For this review, use the dimensioned drawing (mm, ordinates from the lowest corner) and the shaded views. Coordinates: 2 decimals unless noted, no trailing zeros. Order: outer loops, then holes, each group sorted by start corner. A loop starts at its lowest first (then second) coordinate and runs counter-clockwise, first axis right, second up. Notation, with made-up numbers: M 63,20 L 101,20 A19 ccw 101,54 Z; hole C -26,42 d11. An arc over 180 degrees is marked long. Use one line per item in the form item = value. Start each with the question number.
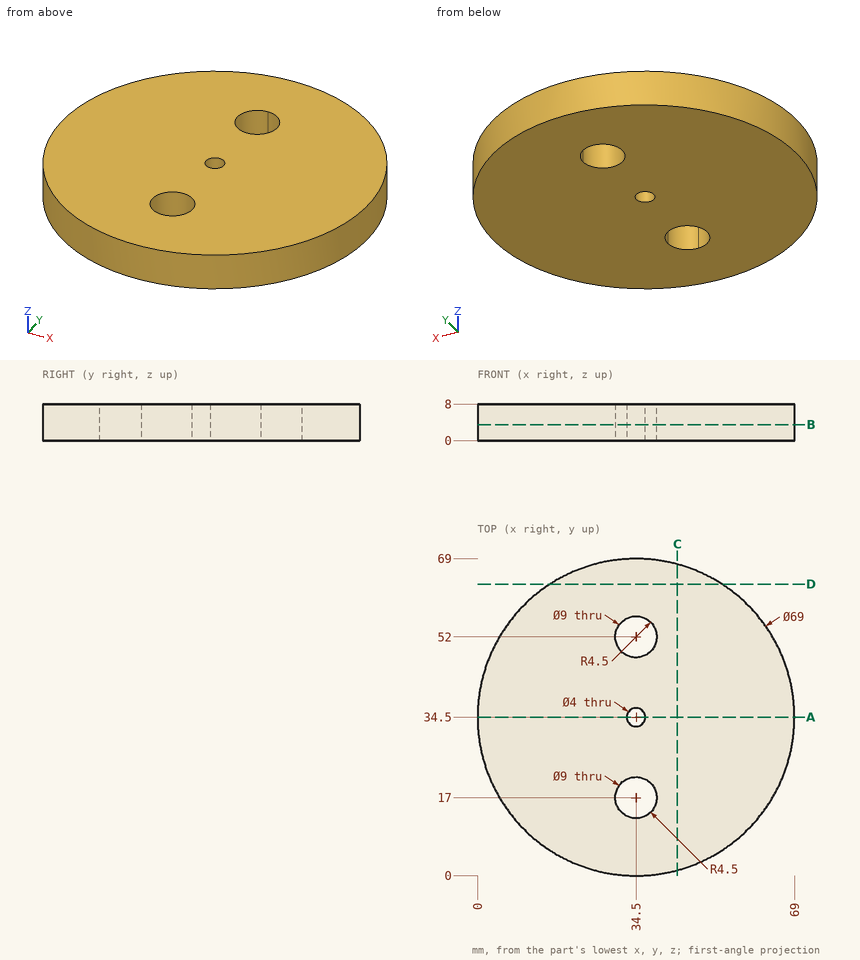
1. Consider section A-A, the plane y = 34.5. Write out the cut boundary in (x, z), plus the area to 3 significant figures.
2. To check wall thickness, follow line 1 (Y direction, x = 34.5, z = 3.75); line 2 (Y direction, x = 37.5, z = 5.5); line 3 (X direction, y = 17, z = 2.75). State the ranges of each line that lie inside material, in increasing order.
3. Consider section C-C, the plane x = 43.5. Write out the cut boundary in (y, z), plus the area to 3 significant figures.
4. Consider section D-D, the plane y = 63.5. Write out the cut boundary in (x, z).
5. Consider section B-B, the plane z = 3.5. Write out the cut boundary in (x, y).
6. For pin 1 Ø3 at (x, z) = (50, 1.5) entering from +Y; pin 2 Ø2 at (x, z) = (51, 1) entering from +Y; pin 3 Ø3 at (x, y) = (34.5, 34.5) entering from +Z; pin 4 Ø4 at (y, z) = (60.5, 4.5) entering from +X, all flat-tipped, find the tip position at first contact; note any pin that passes through.
Answers follow:
q1.outline = M 0,0 L 32.5,0 L 32.5,8 L 0,8 Z; M 36.5,0 L 69,0 L 69,8 L 36.5,8 Z
q1.area = 520 mm²
q2.line_1 = 0 to 12.5, 21.5 to 32.5, 36.5 to 47.5, 56.5 to 69
q2.line_2 = 0.13 to 13.65, 20.35 to 48.65, 55.35 to 68.87
q2.line_3 = 4.77 to 30, 39 to 64.23
q3.outline = M 1.19,0 L 67.81,0 L 67.81,8 L 1.19,8 Z
q3.area = 533 mm²
q4.outline = M 15.81,0 L 53.19,0 L 53.19,8 L 15.81,8 Z
q5.outline = C 34.5,34.5 d69; hole C 34.5,17 d9; hole C 34.5,52 d9; hole C 34.5,34.5 d4
q6.pin_1 = 66.03
q6.pin_2 = 65.32
q6.pin_3 = through
q6.pin_4 = 59.28
